from build123d import *

# Parameters (mm, degrees)
SKETCH_1_R                    = 4
EXTRUDE_1_DEPTH               = 15
SKETCH_2_W                    = 6.467517269
SKETCH_2_H                    = 62.62553055
CUT_EXTRUDE_1_DEPTH           = 55
SKETCH_3_R                    = 5
SKETCH_3_R_2                  = 2.5
CUT_EXTRUDE_2_DEPTH           = 103.877774352
CHAMFER_1_SIZE                = 10
CHAMFER_2_SIZE                = 11
CHAMFER_2_SIZE2               = 7.519269615
FILLET_1_R                    = 5
SKETCH_4_R                    = 2
CUT_EXTRUDE_3_DEPTH           = 103.877774352
SKETCH_5_R                    = 3
CUT_EXTRUDE_4_DEPTH           = 1.5
CUT_EXTRUDE_4_DRAFT           = -33
CUT_EXTRUDE_4_PROFILE_2_DEPTH = 1.5
CUT_EXTRUDE_4_PROFILE_2_DRAFT = -33
CUT_EXTRUDE_4_PROFILE_3_DEPTH = 1.5
CUT_EXTRUDE_4_PROFILE_3_DRAFT = -33
CUT_EXTRUDE_4_PROFILE_4_DEPTH = 1.5
CUT_EXTRUDE_4_PROFILE_4_DRAFT = -33
CUT_EXTRUDE_4_PROFILE_5_DEPTH = 1.5
CUT_EXTRUDE_4_PROFILE_5_DRAFT = -33
CUT_EXTRUDE_4_PROFILE_6_DEPTH = 1.5
CUT_EXTRUDE_4_PROFILE_6_DRAFT = -33
CHAMFER_3_SIZE                = 3


with BuildPart() as part:
    # Эскиз1 → Вытянуть1 (new body)
    with BuildSketch(Plane(origin=(0, 0, 0), x_dir=(0, 0, -1), z_dir=(1, 0, 0))):
        Polygon((-24.418434976, -32.650020726), (-6.60217121, -32.650020726), (-6.60217121, -92.442667507), (35.288487723, -92.442667507), (42.581565024, -60.831663771), (42.581565024, 0.195067042), (-24.418434965, 0.195067042), align=None)
        with Locations((13.784244497, -76.834002497)):
            Circle(SKETCH_1_R, mode=Mode.SUBTRACT)
    extrude(amount=-EXTRUDE_1_DEPTH)

    # Эскиз2 → Вырез-Вытянуть1 (cut, symmetric)
    with BuildSketch(Plane.XY):
        with Locations((-1.770599523, -71.740194192)):
            Rectangle(SKETCH_2_W, SKETCH_2_H)
    extrude(amount=CUT_EXTRUDE_1_DEPTH, both=True, mode=Mode.SUBTRACT)

    # Эскиз3 → Вырез-Вытянуть2 (cut, through all)
    with BuildSketch(Plane.ZY.offset(15)):
        with Locations((8.904690385, -16.227476847)):
            Circle(SKETCH_3_R)
        with Locations((-37.581565054, -16.227476862)):
            Circle(SKETCH_3_R_2)
        with Locations((-24.581565054, -16.227476862)):
            Circle(SKETCH_3_R_2)
    extrude(amount=-CUT_EXTRUDE_2_DEPTH, mode=Mode.SUBTRACT)

    # Фаска1
    chamfer_1_edges = [part.edges().sort_by_distance(p)[0] for p in [
        (-10.002179078, -92.442667507, 6.60217121),
    ]]
    chamfer(chamfer_1_edges, length=CHAMFER_1_SIZE)

    # Фаска2
    chamfer_2_edges = [part.edges().sort_by_distance(p)[0] for p in [
        (-10.002179078, -92.442667507, -35.288487723),
    ]]
    chamfer_2_side = [part.faces().sort_by_distance(p)[0] for p in [
        (-10.002179078, -76.637165639, -38.935026373),
    ]]
    chamfer(chamfer_2_edges, length=CHAMFER_2_SIZE, length2=CHAMFER_2_SIZE2, reference=chamfer_2_side[0])

    # Скругление1
    fillet_1_edges = [part.edges().sort_by_distance(p)[0] for p in [
        (-7.5, -32.650020726, 6.60217121),
    ]]
    fillet(fillet_1_edges, radius=FILLET_1_R)

    # Эскиз4 → Вырез-Вытянуть3 (cut, through all)
    with BuildSketch(Plane.ZY.offset(15)):
        with Locations((-34, -6.080814008)):
            Circle(SKETCH_4_R)
        with Locations((-9, -6.080814008)):
            Circle(SKETCH_4_R)
        with Locations((16, -6.080814008)):
            Circle(SKETCH_4_R)
        with Locations(Location((16, -26.374139717, 0), (0, 0, 180))):
            Circle(SKETCH_4_R)
        with Locations(Location((-9, -26.374139717, 0), (0, 0, 180))):
            Circle(SKETCH_4_R)
        with Locations(Location((-34, -26.374139717, 0), (0, 0, 180))):
            Circle(SKETCH_4_R)
    extrude(amount=-CUT_EXTRUDE_3_DEPTH, mode=Mode.SUBTRACT)


with BuildPart() as cut_extrude_4_tool:
    # Эскиз5 → Вырез-Вытянуть4 (with draft: the straight prism first)
    with BuildSketch(Plane.ZY.offset(15)):
        with Locations((-34, -6.080814008)):
            Circle(SKETCH_5_R)
    extrude(amount=-CUT_EXTRUDE_4_DEPTH)
    # Вырез-Вытянуть4: the draft: its side faces are tilted about the plane it starts from
    cut_extrude_4_sides = [cut_extrude_4_tool.faces().sort_by_distance(p)[0] for p in [
        (-14.25, -6.080814008, -37),
    ]]
    draft(cut_extrude_4_sides, Plane.ZY.offset(15), CUT_EXTRUDE_4_DRAFT)


with BuildPart() as part_1:
    add(part.part)

    # Вырез-Вытянуть4: cut by cut_extrude_4_tool
    add(cut_extrude_4_tool.part, mode=Mode.SUBTRACT)


with BuildPart() as cut_extrude_4_profile_2_tool:
    # Эскиз5 → Вырез-Вытянуть4 profile 2 (with draft: the straight prism first)
    with BuildSketch(Plane.ZY.offset(15)):
        with Locations((-9, -6.080814008)):
            Circle(SKETCH_5_R)
    extrude(amount=-CUT_EXTRUDE_4_PROFILE_2_DEPTH)
    # Вырез-Вытянуть4 profile 2: the draft: its side faces are tilted about the plane it starts from
    cut_extrude_4_profile_2_sides = [cut_extrude_4_profile_2_tool.faces().sort_by_distance(p)[0] for p in [
        (-14.25, -6.080814008, -12),
    ]]
    draft(cut_extrude_4_profile_2_sides, Plane.ZY.offset(15), CUT_EXTRUDE_4_PROFILE_2_DRAFT)


with BuildPart() as part_2:
    add(part_1.part)

    # Вырез-Вытянуть4 profile 2: cut by cut_extrude_4_profile_2_tool
    add(cut_extrude_4_profile_2_tool.part, mode=Mode.SUBTRACT)


with BuildPart() as cut_extrude_4_profile_3_tool:
    # Эскиз5 → Вырез-Вытянуть4 profile 3 (with draft: the straight prism first)
    with BuildSketch(Plane.ZY.offset(15)):
        with Locations((16, -6.080814008)):
            Circle(SKETCH_5_R)
    extrude(amount=-CUT_EXTRUDE_4_PROFILE_3_DEPTH)
    # Вырез-Вытянуть4 profile 3: the draft: its side faces are tilted about the plane it starts from
    cut_extrude_4_profile_3_sides = [cut_extrude_4_profile_3_tool.faces().sort_by_distance(p)[0] for p in [
        (-14.25, -6.080814008, 13),
    ]]
    draft(cut_extrude_4_profile_3_sides, Plane.ZY.offset(15), CUT_EXTRUDE_4_PROFILE_3_DRAFT)


with BuildPart() as part_3:
    add(part_2.part)

    # Вырез-Вытянуть4 profile 3: cut by cut_extrude_4_profile_3_tool
    add(cut_extrude_4_profile_3_tool.part, mode=Mode.SUBTRACT)


with BuildPart() as cut_extrude_4_profile_4_tool:
    # Эскиз5 → Вырез-Вытянуть4 profile 4 (with draft: the straight prism first)
    with BuildSketch(Plane.ZY.offset(15)):
        with Locations((16, -26.374139717)):
            Circle(SKETCH_5_R)
    extrude(amount=-CUT_EXTRUDE_4_PROFILE_4_DEPTH)
    # Вырез-Вытянуть4 profile 4: the draft: its side faces are tilted about the plane it starts from
    cut_extrude_4_profile_4_sides = [cut_extrude_4_profile_4_tool.faces().sort_by_distance(p)[0] for p in [
        (-14.25, -26.374139717, 13),
    ]]
    draft(cut_extrude_4_profile_4_sides, Plane.ZY.offset(15), CUT_EXTRUDE_4_PROFILE_4_DRAFT)


with BuildPart() as part_4:
    add(part_3.part)

    # Вырез-Вытянуть4 profile 4: cut by cut_extrude_4_profile_4_tool
    add(cut_extrude_4_profile_4_tool.part, mode=Mode.SUBTRACT)


with BuildPart() as cut_extrude_4_profile_5_tool:
    # Эскиз5 → Вырез-Вытянуть4 profile 5 (with draft: the straight prism first)
    with BuildSketch(Plane.ZY.offset(15)):
        with Locations((-9, -26.374139717)):
            Circle(SKETCH_5_R)
    extrude(amount=-CUT_EXTRUDE_4_PROFILE_5_DEPTH)
    # Вырез-Вытянуть4 profile 5: the draft: its side faces are tilted about the plane it starts from
    cut_extrude_4_profile_5_sides = [cut_extrude_4_profile_5_tool.faces().sort_by_distance(p)[0] for p in [
        (-14.25, -26.374139717, -12),
    ]]
    draft(cut_extrude_4_profile_5_sides, Plane.ZY.offset(15), CUT_EXTRUDE_4_PROFILE_5_DRAFT)


with BuildPart() as part_5:
    add(part_4.part)

    # Вырез-Вытянуть4 profile 5: cut by cut_extrude_4_profile_5_tool
    add(cut_extrude_4_profile_5_tool.part, mode=Mode.SUBTRACT)


with BuildPart() as cut_extrude_4_profile_6_tool:
    # Эскиз5 → Вырез-Вытянуть4 profile 6 (with draft: the straight prism first)
    with BuildSketch(Plane.ZY.offset(15)):
        with Locations((-34, -26.374139717)):
            Circle(SKETCH_5_R)
    extrude(amount=-CUT_EXTRUDE_4_PROFILE_6_DEPTH)
    # Вырез-Вытянуть4 profile 6: the draft: its side faces are tilted about the plane it starts from
    cut_extrude_4_profile_6_sides = [cut_extrude_4_profile_6_tool.faces().sort_by_distance(p)[0] for p in [
        (-14.25, -26.374139717, -37),
    ]]
    draft(cut_extrude_4_profile_6_sides, Plane.ZY.offset(15), CUT_EXTRUDE_4_PROFILE_6_DRAFT)


with BuildPart() as part_6:
    add(part_5.part)

    # Вырез-Вытянуть4 profile 6: cut by cut_extrude_4_profile_6_tool
    add(cut_extrude_4_profile_6_tool.part, mode=Mode.SUBTRACT)

    # Фаска3
    chamfer_3_edges = [part_6.edges().sort_by_distance(p)[0] for p in [
        (-15, 0.195067042, -9.08156503),
    ]]
    chamfer(chamfer_3_edges, length=CHAMFER_3_SIZE)


solid = part_6.part
Build history of the part. All positions in model axes, mm. A direction names the side the tool comes from. Round coordinates to 2 decimals unless told otherwise and drop trailing zeros. Write each loop counter-clockwise with the first axis right and the second up, starting at its lowest first coordinate (ties: lowest second). Pieces come first, ordered by that corner, then holes. Notation, with made-up numbers: M -6.75,22.25 L 0.25,22.25 A12 ccw 0.25,39.25 Z; hole C 28.25,16 d10. An arc over 180 degrees is marked long. Answer as a JSON object with one key per item and string values. Group by question number.
(1) Cut at A-A (z = 16). Give the number of separate pieces and of enclosed holes in the cut face, and give its area (3 significant figures).
(2) Cut at D-D (y = -58). Give the cut face in (x, z), and give its area (3 significant figures).
(3) Cut at C-C (z = -13.5). Give the cut face in (x, y), and give its area (4 significant figures).
(4) Flat gauge pins, fed straight in: pin 1 (4 mm diameter, centred on x = -13.5, y = -77.5, fed in from -Z); pin 2 (15 mm diameter, centred on y = -54.5, z = -25, fed in from +X); pin 3 (5 mm diameter, centred on x = -11, y = -63, fed in from +Z). Where does each tip first touch, or does it go through?
(5) Drill centre lines: L1, parallel to Y at x = -7, z = 16; L2, parallel to Y at x = -4, z = -34; L3, parallel to Y at x = -8, z = 20. Where is each one in solid material? Low to high.
(6) Mould opens along Z. For faces 4 (the flat face through (-9, -60, 6.602)), 5 (the flat face through (-9.93, -71.42, -40.14)), 6 (the cylindrical face through (-7.6, -21.11, 7.82)), 7 (the cylindrical face through (-6.844, -6.847, -32.153)) say: pulls with the +Z half, pulls with the -Z half, needs draft (parallel to the pull), parting line crosses it, or undercut.
(7) Which spindle directions (+Z, -Z, +X, -X, +Y, -Y) get a long thin tool onto all of the face, cutting with end or side? Do faces 1 (the cylindrical face through (-6.844, -28.357, 16.26)), 2 (the flat face through (-3, -40.427, -18)), 3 (the flat face through (-7, -32.65, 18)). Say none if no direction does.
Responses:
{
 "1": {"separate pieces": "3", "enclosed holes": "0", "area": "365 mm2"},
 "2": {"outline": "M -15,-42.58 L -5,-42.58 L -5,6.6 L -15,6.6 Z", "area": "492 mm2"},
 "3": {"outline": "M -15,-92.44 L -5,-92.44 L -5,-80.82 L -15,-80.82 Z; M -15,-72.84 L -5,-72.84 L -5,-40.43 L 0,-40.43 L 0,0.2 L -12,0.2 L -15,-2.8 Z", "area": "1,045 mm2"},
 "4": {"pin 1": "stops at z = -39.2", "pin 2": "stops at x = -5", "pin 3": "stops at z = 6.6"},
 "5": {"L1": "y = -32.65 to -28.37, -24.37 to -8.08, -4.08 to 0.2", "L2": "y = -40.43 to -28.37, -24.37 to -8.08, -4.08 to 0.2", "L3": "y = -32.65 to 0.2"},
 "6": {"face 4": "pulls with the +Z half", "face 5": "pulls with the -Z half", "face 6": "undercut", "face 7": "undercut"},
 "7": {"face 1": "+X, -X", "face 2": "+Z, -Z, +X, -Y", "face 3": "+Z, +X, -X, -Y"}
}
